from build123d import *

# Parameters (mm, degrees)
DODANIE_WYCI_GNI_CIE1_DEPTH = 15
ZAOKR_GLENIE1_R             = 2
OTWORY_USTALAJ_CE_6_0MM3_D  = 6
ZAOKR_GLENIE2_R             = 1


with BuildPart() as part:
    # Szkic1 → Dodanie-wyciągnięcie1 (new body)
    with BuildSketch(Plane.XY):
        with BuildLine():
            Line((-29, 0), (-29, 6.5))
            Line((-29, 6.5), (-17, 6.5))
            ThreePointArc((-17, 6.5), (-14.071067812, 13.571067812), (-7, 16.5))
            Line((-7, 16.5), (7, 16.5))
            ThreePointArc((7, 16.5), (14.071067812, 13.571067812), (17, 6.5))
            Line((17, 6.5), (29, 6.5))
            Line((29, 6.5), (29, 0))
            Line((29, 0), (11.5, 0))
            ThreePointArc((11.5, 0), (0, 11.5), (-11.5, 0))
            Line((-11.5, 0), (-29, 0))
        make_face()
    extrude(amount=DODANIE_WYCI_GNI_CIE1_DEPTH)

    # Zaokrąglenie1
    zaokr_glenie1_edges = [part.edges().sort_by_distance(p)[0] for p in [
        (-17, 6.5, 7.5),
        (17, 6.5, 7.5),
    ]]
    fillet(zaokr_glenie1_edges, radius=ZAOKR_GLENIE1_R)

    # Otwory ustalające Ø6.0mm3 (through all)
    with Locations(Plane(origin=(0, 6.5, 0), x_dir=(1, 0, 0), z_dir=(0, 1, 0))):
        with Locations((-23.5, -7.5)):
            otwory_ustalaj_ce_6_0mm3 = Hole(OTWORY_USTALAJ_CE_6_0MM3_D / 2)

    # Lustro1: Otwory ustalające Ø6.0mm3 across plane
    add(otwory_ustalaj_ce_6_0mm3.mirror(Plane(origin=(0, 0, 0), x_dir=(0, 0, 1), z_dir=(1, 0, 0))), mode=Mode.SUBTRACT)

    # Zaokrąglenie2
    zaokr_glenie2_edges = [part.edges().sort_by_distance(p)[0] for p in [
        (29, 6.5, 7.5),
        (-29, 6.5, 7.5),
    ]]
    fillet(zaokr_glenie2_edges, radius=ZAOKR_GLENIE2_R)


solid = part.part
For this review, take the finished solid that the model builds, in its own axes (mm). A direction names the side the tool comes from. Round coordinates to 2 decimals unless told otherwise and drop trailing zeros. Write each loop counter-clockwise with the first axis right and the second up, starting at its lowest first coordinate (ties: lowest second). Pieces come first, ordered by that corner, then holes. Notation, with made-up numbers: (69.5, 82.5) -> (104.5, 82.5) arc R17 ccw to (104.5, 114.5) -> close; hole circle Ø3 at (-0.5, 5). An arc over 180 degrees is marked (long way). Use CSV: the item, a comma, the result in double quotes.
(1) Consider section A-A, the plane z = 7.5. Give the boundary of the cut face in (x, y).
Computed values:
outline,"(-29, 0) -> (-26.5, 0) -> (-26.5, 6.5) -> (-28, 6.5) arc R1 ccw to (-29, 5.5) -> close; (-20.5, 0) -> (-11.5, 0) arc R11.5 cw to (11.5, 0) -> (20.5, 0) -> (20.5, 6.5) -> (18.83, 6.5) arc R2 cw to (16.86, 8.17) arc R10 ccw to (7, 16.5) -> (-7, 16.5) arc R10 ccw to (-16.86, 8.17) arc R2 cw to (-18.83, 6.5) -> (-20.5, 6.5) -> close; (26.5, 0) -> (29, 0) -> (29, 5.5) arc R1 ccw to (28, 6.5) -> (26.5, 6.5) -> close"
(2) Clearance check with flat-ended pins moving along their axes: P1, Ø5, axis at x = -0.5, z = 9, coming from the -Y side; P2, Ø3, axis at x = 23.5, z = 5.5, coming from the +Y side; P3, Ø2, axis at x = 8, z = 6, coming from the -Y side. State where each tip first meets the part, or that it passes through.
Computed values:
P1,"y = 11.1"
P2,"y = 6.5"
P3,"y = 7.16"
(3) For faces 5 (the face through (20, 6.5, 7)), 6 (the face through (0, 12, 0)), list the 3-axis set-ups (+Z, -Z, +X, -X, +Y, -Y) from which the entire face can be reached by the end or side of a thin tool; tool diameter is ignored.
Computed values:
face 5,"+Z, -Z, +X, +Y"
face 6,"-Z, +X, -X, +Y, -Y"
(4) Consider section D-D, the plane z = 14.25. Give the boundary of the cut face in (x, y), plus the area to 3 significant figures.
Computed values:
outline,"(-29, 0) -> (-11.5, 0) arc R11.5 cw to (11.5, 0) -> (29, 0) -> (29, 5.5) arc R1 ccw to (28, 6.5) -> (18.83, 6.5) arc R2 cw to (16.86, 8.17) arc R10 ccw to (7, 16.5) -> (-7, 16.5) arc R10 ccw to (-16.86, 8.17) arc R2 cw to (-18.83, 6.5) -> (-28, 6.5) arc R1 ccw to (-29, 5.5) -> close"
area,"467 mm²"
(5) Draft analysis for pull direction X (two halves, no side actions). For faces 1 (the face through (-17.556, 6.96, 7.605)), 2 (the face through (29, 3, 7)), 3 (the face through (0.253, 11.497, 7.395)), 4 (the face through (-20, 6.5, 7)), state which applies: +X half, -X half, draft (parallel to the pull), parting line (faces both ways), or undercut.
Computed values:
face 1,"-X half"
face 2,"+X half"
face 3,"undercut"
face 4,"draft"
(6) Consider section B-B, the plane x = -23.5. Give the boundary of the cut face in (y, z).
Computed values:
outline,"(0, 0) -> (6.5, 0) -> (6.5, 4.5) -> (0, 4.5) -> close; (0, 10.5) -> (6.5, 10.5) -> (6.5, 15) -> (0, 15) -> close"
(7) To check wall thickness, follow L1, parallel to Z at x = 23.5, y = 4.5; L2, parallel to X at y = 4.25, z = 8.25; L3, parallel to X at y = 5.25, z = 8.5. State the ranges of each line that lie inside material, in increasing order. Write a range as [from, to].
Computed values:
L1,"[0, 4.5], [10.5, 15]"
L2,"[-29, -26.4], [-20.6, -10.69], [10.69, 20.6], [26.4, 29]"
L3,"[-29, -26.33], [-20.67, -10.23], [10.23, 20.67], [26.33, 29]"
(8) Consider section C-C, the plane y = 10.25. Give the boundary of the cut face in (x, z).
Computed values:
outline,"(-16.27, 0) -> (-5.21, 0) -> (-5.21, 15) -> (-16.27, 15) -> close; (5.21, 0) -> (16.27, 0) -> (16.27, 15) -> (5.21, 15) -> close"
